Design review of the part built by this model. Coordinates are the model's own, in mm. A direction names the side the tool comes from. Coordinates: 2 decimals unless noted, no trailing zeros. Write each loop counter-clockwise with the first axis right and the second up, starting at its lowest first coordinate (ties: lowest second). Pieces come first, ordered by that corner, then holes.
Q1. Take a section at D-D, the plane x = -33. Write out the cut boundary in (y, z), plus the area to 3 significant figures.
Q2. For faces 1 (the flat face through (-20, 5, 30)), 2 (the flat face through (-15, 10, 30)), 3 (the flat face through (-30, 30, 10)), list the 3-axis set-ups (+Z, -Z, +X, -X, +Y, -Y) from which the entire face can be reached by the end or side of a thin tool; tool diameter is ignored.
Q3. For pin 1 Ø12 at (y, z) = (28, 7) entering from -X; pin 2 Ø5 at (y, z) = (5, 25.5) entering from -X; pin 3 Ø6 at (x, z) = (-38.5, 11.5) entering from +Y, all flat-tipped, find the tip position at first contact; note any pin that passes through.
Q4. For L1, parallel to X at y = 5, z = 23.5; L2, parallel to Z at x = -24, y = 35; L3, parallel to Y at x = -13, z = 35.5, list the stretches that pass through material, from the lowest coordinate up.
Q5. Take a section at A-A, the plane z = 25. Write out the cut boundary in (x, y).
Q6. Take a section at C-C, the plane x = -23.5. Write out the cut boundary in (y, z), plus the area to 3 significant figures.
Q7. Take a section at B-B, the plane y = 29.5. Write out the cut boundary in (x, z).
from build123d import *

# Parameters (mm, degrees)
F0_W     = 40
F0_H     = 40
F1_DEPTH = 10
F2_W     = 40
F2_H     = 20
F3_DEPTH = 20
F4_W     = 20
F4_H     = 20
F5_DEPTH = 20
F6_W     = 10
F6_H     = 20
F7_DEPTH = 10


with BuildPart() as f1:
    # F0 (on Right) → F1 (new body)
    with BuildSketch(Plane.YZ):
        with Locations((20, 20)):
            Rectangle(F0_W, F0_H)
    extrude(amount=-F1_DEPTH)

    # F2 (on face) → F3 (join)
    with BuildSketch(Plane(origin=(-10, 0, 0), x_dir=(0, -1, 0), z_dir=(-1, 0, 0))):
        with Locations((-20, 10)):
            Rectangle(F2_W, F2_H)
    extrude(amount=F3_DEPTH)

    # F4 (on face) → F5 (join)
    with BuildSketch(Plane(origin=(-30, 0, 0), x_dir=(0, -1, 0), z_dir=(-1, 0, 0))):
        with Locations((-10, 10)):
            Rectangle(F4_W, F4_H)
    extrude(amount=F5_DEPTH)

    # F6 (on face) → F7 (join)
    with BuildSketch(Plane(origin=(-10, 0, 0), x_dir=(0, -1, 0), z_dir=(-1, 0, 0))):
        with Locations((-5, 30)):
            Rectangle(F6_W, F6_H)
    extrude(amount=F7_DEPTH)


solid = f1.part
Responses:
1. outline: (0, 0) - (20, 0) - (20, 20) - (0, 20) - close
1. area: 400 mm2
2. face 1: +Z, -X, +Y, -Y
2. face 2: +Z, -X, +Y
2. face 3: +Z, -Z, -X, +Y
3. pin 1: stops at x = -30
3. pin 2: stops at x = -20
3. pin 3: stops at y = 20
4. L1: x = -20 to 0
4. L2: z = 0 to 20
4. L3: y = 0 to 10
5. outline: (-20, 0) - (0, 0) - (0, 40) - (-10, 40) - (-10, 10) - (-20, 10) - close
6. outline: (0, 0) - (40, 0) - (40, 20) - (0, 20) - close
6. area: 800 mm2
7. outline: (-30, 0) - (0, 0) - (0, 40) - (-10, 40) - (-10, 20) - (-30, 20) - close
